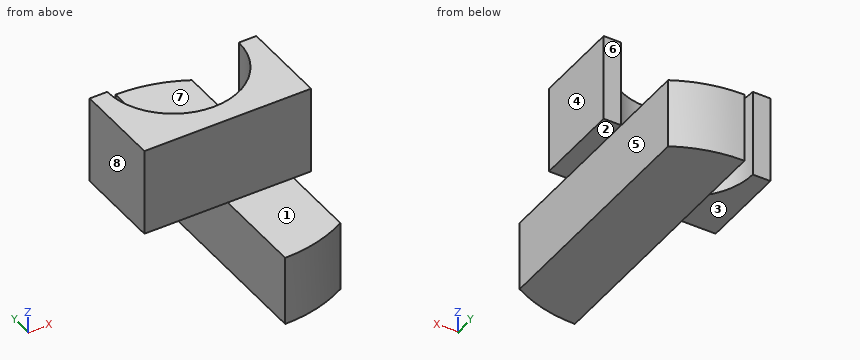
from build123d import *

# Parameters (mm, degrees)
EXTRUDE_1_DEPTH = 8
EXTRUDE_2_DEPTH = 10


with BuildPart() as part:
    # 草图1 → 凸台-拉伸1 (new body)
    with BuildSketch(Plane.XY):
        with BuildLine():
            Line((7.5, -13.564659966), (7.5, 13.564659966))
            ThreePointArc((7.5, 13.564659966), (3.872839431, 15.008368157), (0, 15.5))
            Line((0, 15.5), (0, -15.5))
            ThreePointArc((0, -15.5), (3.872839431, -15.008368157), (7.5, -13.564659966))
        make_face()
    extrude(amount=EXTRUDE_1_DEPTH)

    # 草图3 → 凸台-拉伸2 (add)
    with BuildSketch(Plane.XY.offset(8)):
        Polygon((7.5, -2.5), (7.5, -5), (9.5, -5), (9.5, 5), (7.5, 5), align=None)
        with BuildLine():
            Line((0, -2.5), (0, -5))
            Line((0, -5), (7.5, -5))
            Line((7.5, -5), (7.5, -2.5))
            Line((7.5, -2.5), (7.5, 5))
            ThreePointArc((7.5, 5), (5.303300859, -0.303300859), (0, -2.5))
        make_face()
        with BuildLine():
            Line((-7.5, 5), (-7.5, -2.5))
            Line((-7.5, -2.5), (-7.5, -5))
            Line((-7.5, -5), (0, -5))
            Line((0, -5), (0, -2.5))
            ThreePointArc((0, -2.5), (-5.303300859, -0.303300859), (-7.5, 5))
        make_face()
        Polygon((-9.5, 5), (-7.5, 5), (-7.5, -2.5), (-7.5, -5), (-9.5, -5), align=None)
    extrude(amount=EXTRUDE_2_DEPTH)


solid = part.part
Part model, mm, in its own coordinate system. Face numbers are marked on the shaded views. A direction names the side the tool comes from. Give positions to 0.01 mm unless a question says otherwise; leave off trailing zeros. Loops run counter-clockwise (first coordinate to the right, second up) from the corner with the lowest first, then second, coordinate; pieces in that order, holes last. Notation, with made-up numbers: (80.5, -32.5) -> (111.5, -32.5) arc R9 cw to (111.5, -15.5) -> close; hole circle Ø6 at (59.5, 56). An arc over 180 degrees is marked (long way). Write each question's results on one line, items separated by ' | '. Start each with the question number.
Q1. Which spindle directions (+Z, -Z, +X, -X, +Y, -Y) get a long thin tool onto all of the face, cutting with end or side? Do the marked faces 1, 2, 3 and 4. Say none if no direction does.
Q2. Wall check: L1, parallel to Z at x = -5.75, y = -3; L2, parallel to X at y = -5, z = 3.75; L3, parallel to Z at x = 0.25, y = -11.5. Give the ranges that are in metal, low to high.
Q3. Pin check, flat tips, straight feed: P1, Ø0.6, axis at x = -8, z = 12.5, coming from the +Y side; P2, Ø3, axis at x = -7.5, z = 9.5, coming from the -Y side; P3, Ø6, axis at x = 5, y = -9, coming from the +Z side. Stop position of each tip, or through.
Q4. Pull direction X, two halves, no side cores. Call the marked faces 5, 6, 7 and 8: +X half, -X half, draft (parallel to the pull), parting line (faces both ways), or undercut.
Q5. Band-saw the part on D-D on y = 7. List the corners of the cut face in (x, z).
Q6. Band-saw the part on C-C on x = 4.5. List the corners of the cut face in (y, z).
Q7. Band-saw the part on B-B on z = 12.75. List the corners of the cut face in (x, y).
Q8. Band-saw the part on A-A on y = -1. List the corners of the cut face in (x, z).
Results are:
1) face 1: +Z, +X, -X, -Y | face 2: -Z, +X, +Y, -Y | face 3: -Z, -X, +Y, -Y | face 4: +Z, -Z, +X, +Y, -Y
2) L1: z = 8 to 18 | L2: x = 0 to 7.5 | L3: z = 0 to 8
3) P1: stops at y = 5 | P2: stops at y = -5 | P3: stops at z = 8
4) face 5: +X half | face 6: draft | face 7: undercut | face 8: -X half
5) outline: (0, 0) -> (7.5, 0) -> (7.5, 8) -> (0, 8) -> close
6) outline: (-14.83, 0) -> (14.83, 0) -> (14.83, 8) -> (-1, 8) -> (-1, 18) -> (-5, 18) -> (-5, 8) -> (-14.83, 8) -> close
7) outline: (-9.5, -5) -> (9.5, -5) -> (9.5, 5) -> (7.5, 5) arc R7.5 cw to (-7.5, 5) -> (-9.5, 5) -> close
8) outline: (-9.5, 8) -> (-4.5, 8) -> (-4.5, 18) -> (-9.5, 18) -> close; (0, 0) -> (7.5, 0) -> (7.5, 8) -> (9.5, 8) -> (9.5, 18) -> (4.5, 18) -> (4.5, 8) -> (0, 8) -> close
